Geometry: final body of the model. Coordinates: model frame, mm. A direction names the side the tool comes from. Give positions to 0.01 mm unless a question says otherwise; leave off trailing zeros. Write each loop counter-clockwise with the first axis right and the second up, starting at its lowest first coordinate (ties: lowest second). Pieces come first, ordered by that corner, then holes. Notation, with made-up numbers: (-5.75, 38) -> (23.25, 38) arc R26 cw to (23.25, 62) -> close; hole circle Ø11 at (38, 83.25). An arc over 180 degrees is marked (long way). Answer as a JSON object with one key per item and string values. Group by question number.
(1) Section query B-B on x = 0. Output: boundary loops of the cut face in (y, z), plus the area to 3 significant figures.
(2) Contact query for flat-ended pins moving along their axis: pin 1 Ø1.8 at (x, z) = (0, 0) entering from +Y; pin 2 Ø2 at (x, z) = (-2, -6) entering from +Y; pin 3 Ø1 at (x, y) = (-9.5, 2.5) entering from +Z; pin 4 Ø4.5 at (x, z) = (-9, -6) entering from +Y. Output: stop coordinate, or through.
(3) Draft query along X for faces 4 (the face through (9, 6, -0.4)), 5 (the face through (-6.74, 6, -8)). Return one class per face: +X half, -X half, draft (parallel to the pull), parting line (faces both ways), or undercut.
(4) Section query A-A on y = 1.25. Output: boundary loops of the cut face in (x, z), plus the area to 3 significant figures.
(5) Section query C-C on z = 0. Output: boundary loops of the cut face in (x, y), plus the area to 3 significant figures.
(6) Set-up query: faces 1 (the face through (-8, 11.7, -6)), 2 (the face through (-9.6, 5.6, -0.4)), 3 (the face through (-8.505, 5.565, -3.508)). Return all of +Z, -Z, +X, -X, +Y, -Y with unobstructed straight access to the full face (end or side cutting, diameter ignored); none if empty.
(7) Material intervals for probe 1 along Z at (x, y) = (0, 8.5); probe 2 along Y at (x, z) = (3, 7); probe 3 along X at (y, z) = (1, 2.75), sorted ascending.
from build123d import *

# Parameters (mm, degrees)
SKETCH013_R     = 1.5
POCKET001_DEPTH = 23.8
PAD008_DEPTH    = 10.5
PAD009_DEPTH    = 12.1
SKETCH047_W     = 0.8
SKETCH047_H     = 0.8
POCKET005_DEPTH = 10.5


with BuildPart() as part:
    # Sketch007 → Revolution (revolve)
    with BuildSketch(Plane.XY):
        Polygon((0, 10.9), (0.84, 10.9), (2.52, 12.3), (5.88, 9.5), (7.56, 10.9), (8.4, 10.9), (8.4, 0.4), (7.56, 0.4), (5.88, -1), (2.52, 1.8), (0.84, 0.4), (0, 0.4), align=None)
    revolve(axis=Axis((0, 0, 0), (0, 1, 0)))

    # Sketch013 → Pocket001 (cut)
    with BuildSketch(Plane.XZ.offset(1)):
        Circle(SKETCH013_R)
    extrude(amount=-POCKET001_DEPTH, mode=Mode.SUBTRACT)

    # Sketch023 → Pad008 (join)
    with BuildSketch(Plane.XZ.offset(-0.4)):
        with BuildLine():
            Line((-5.939697, -9.2), (10.070471, -9.2))
            Line((10.070471, -9.2), (10.070471, -0.4))
            Line((10.070471, -0.4), (8.390471, -0.4))
            ThreePointArc((-5.939697, -5.939697), (3.028801, -7.834945), (8.390471, -0.4))
            Line((-5.939697, -5.939697), (-5.939697, -9.2))
        make_face()
    extrude(amount=-PAD008_DEPTH)

    # Sketch024 → Pad009 (join)
    with BuildSketch(Plane.XZ.offset(0.4)):
        with BuildLine():
            Line((-10.08, -0.4), (-10.08, -9.2))
            Line((-10.08, -9.2), (-5.939697, -9.2))
            Line((-5.939697, -8.4), (-5.939697, -9.2))
            Line((-6.739697, -8.4), (-5.939697, -8.4))
            Line((-6.739697, -8.4), (-6.739697, -6.262307))
            ThreePointArc((-9.1913, -0.4), (-8.487687, -3.549531), (-6.739697, -6.262307))
            Line((-9.1913, -0.4), (-10.08, -0.4))
        make_face()
    extrude(amount=-PAD009_DEPTH)

    # Sketch047 → Pocket005 (cut)
    with BuildSketch(Plane.XZ.offset(0.4)):
        with Locations((-6.339697, -8.8)):
            Rectangle(SKETCH047_W, SKETCH047_H)
    extrude(amount=-POCKET005_DEPTH, mode=Mode.SUBTRACT)


solid = part.part
Answer list:
{
 "1": {"outline": "(-1, -5.88) -> (0.4, -7.56) -> (0.4, -9.2) -> (10.9, -9.2) -> (10.9, -7.56) -> (9.5, -5.88) -> (12.3, -2.52) -> (11.45, -1.5) -> (0.95, -1.5) -> (1.8, -2.52) -> close; (-1, 5.88) -> (1.8, 2.52) -> (0.95, 1.5) -> (11.45, 1.5) -> (12.3, 2.52) -> (9.5, 5.88) -> (10.9, 7.56) -> (10.9, 8.4) -> (0.4, 8.4) -> (0.4, 7.56) -> close", "area": "153 mm2"},
 "2": {"pin 1": "through", "pin 2": "y = 10.7", "pin 3": "z = -0.4", "pin 4": "y = 11.7"},
 "3": {"face 4": "draft", "face 5": "undercut"},
 "4": {"outline": "(-10.08, -9.2) -> (-6.74, -9.2) -> (-6.74, -6.26) arc R9.2 cw to (-9.19, -0.4) -> (-10.08, -0.4) -> close; (-5.94, -9.2) -> (10.07, -9.2) -> (10.07, -0.4) -> (8.39, -0.4) arc R8.4 ccw (long way) to (-5.94, -5.94) -> close; circle Ø3.72 at (0, 0); hole circle Ø6.36 at (0, 0); hole circle Ø3 at (0, 0)", "area": "259 mm2"},
 "5": {"outline": "(-8.4, 0.4) -> (-7.56, 0.4) -> (-5.88, -1) -> (-2.52, 1.8) -> (-1.5, 0.95) -> (-1.5, 11.45) -> (-2.52, 12.3) -> (-5.88, 9.5) -> (-7.56, 10.9) -> (-8.4, 10.9) -> close; (1.5, 0.95) -> (2.52, 1.8) -> (5.88, -1) -> (7.56, 0.4) -> (8.4, 0.4) -> (8.4, 10.9) -> (7.56, 10.9) -> (5.88, 9.5) -> (2.52, 12.3) -> (1.5, 11.45) -> close", "area": "145 mm2"},
 "6": {"face 1": "+Z, -Z, -X, +Y", "face 2": "+Z, -X, +Y, -Y", "face 3": "+Y, -Y"},
 "7": {"probe 1": "-9.2 to -1.5, 1.5 to 8.4", "probe 2": "0.4 to 10.9", "probe 3": "-7.94 to -2.13, 2.13 to 7.94"}
}
